from build123d import *

# Parameters (mm, degrees)
SKETCH1_R           = 9.25
SKETCH1_R_2         = 6.5
BOSS_EXTRUDE1_DEPTH = 62.5
BOSS_EXTRUDE2_START = -15
SKETCH3_R           = 12.5
SKETCH3_R_2         = 6.5
BOSS_EXTRUDE2_DEPTH = 15
BOSS_EXTRUDE3_START = 2.51
SKETCH4_R           = 9.25
SKETCH4_R_2         = 6.5
BOSS_EXTRUDE3_DEPTH = 2.51
BOSS_EXTRUDE4_START = 2.51
SKETCH5_R           = 12.5
SKETCH5_R_2         = 9.25
BOSS_EXTRUDE4_DEPTH = 2.51
CUT_EXTRUDE1_START  = -2.51
SKETCH6_R           = 12.5
SKETCH6_R_2         = 6.5
CUT_EXTRUDE1_DEPTH  = 2.51


with BuildPart() as part:
    # Sketch1 → Boss-Extrude1 (new body)
    with BuildSketch(Plane(origin=(0, 0, 0), x_dir=(1, 0, 0), z_dir=(0, 1, 0))):
        with Locations(Location((0, 0, 0), (0, 0, 270))):
            Circle(SKETCH1_R)
        with Locations(Location((0, 0, 0), (0, 0, 270))):
            Circle(SKETCH1_R_2, mode=Mode.SUBTRACT)
    extrude(amount=BOSS_EXTRUDE1_DEPTH)

    # Sketch3 → Boss-Extrude2 (add)
    with BuildSketch(Plane(origin=(0, 62.5, 0), x_dir=(1, 0, 0), z_dir=(0, 1, 0)).offset(BOSS_EXTRUDE2_START)):
        with Locations(Location((0, 0, 0), (0, 0, 270))):
            Circle(SKETCH3_R)
        with Locations(Location((0, 0, 0), (0, 0, 270))):
            Circle(SKETCH3_R_2, mode=Mode.SUBTRACT)
    extrude(amount=BOSS_EXTRUDE2_DEPTH)

    # Sketch4 → Boss-Extrude3 (add)
    with BuildSketch(Plane.XZ.offset(BOSS_EXTRUDE3_START)):
        with Locations(Location((0, 0, 0), (0, 0, 270))):
            Circle(SKETCH4_R)
        with Locations(Location((0, 0, 0), (0, 0, 270))):
            Circle(SKETCH4_R_2, mode=Mode.SUBTRACT)
    extrude(amount=-BOSS_EXTRUDE3_DEPTH)

    # Sketch5 → Boss-Extrude4 (add)
    with BuildSketch(Plane.XZ.offset(-47.5).offset(BOSS_EXTRUDE4_START)):
        with Locations(Location((0, 0, 0), (0, 0, 90))):
            Circle(SKETCH5_R)
        with Locations(Location((0, 0, 0), (0, 0, 270))):
            Circle(SKETCH5_R_2, mode=Mode.SUBTRACT)
    extrude(amount=-BOSS_EXTRUDE4_DEPTH)

    # Sketch6 → Cut-Extrude1 (cut)
    with BuildSketch(Plane(origin=(0, 62.5, 0), x_dir=(1, 0, 0), z_dir=(0, 1, 0)).offset(CUT_EXTRUDE1_START)):
        with Locations(Location((0, 0, 0), (0, 0, 270))):
            Circle(SKETCH6_R)
        with Locations(Location((0, 0, 0), (0, 0, 90))):
            Circle(SKETCH6_R_2, mode=Mode.SUBTRACT)
    extrude(amount=CUT_EXTRUDE1_DEPTH, mode=Mode.SUBTRACT)


solid = part.part
Build history of the part. All positions in model axes, mm. A direction names the side the tool comes from. Round coordinates to 2 decimals unless told otherwise and drop trailing zeros. Loops run counter-clockwise (first coordinate to the right, second up) from the corner with the lowest first, then second, coordinate; pieces in that order, holes last. Notation, with made-up numbers: (-29, 65.5) -> (-25, 65.5) arc R27 cw to (-25, 87.5) -> close; hole circle Ø5 at (39, 36.5). An arc over 180 degrees is marked (long way). One line per item, written item: value. Start each with the question number.
Q1. Probe line 1 along Z through (x, y) = (0, 34.5); line 2 along X through (y, z) = (50.5, -0.25). List the from-to ranges inside material, lowest first.
Q2. Cut at A-A on x = 0. List the corners of the cut face in (y, z), plus the area to 3 significant figures.
Q3. Drop flat-ended pins along their axis: pin 1 Ø12 at (y, z) = (8.5, -1.5) entering from +X; pin 2 Ø12 at (y, z) = (28, 0) entering from -X; pin 3 Ø8 at (x, y) = (-5.5, 12) entering from -Z. Give the stop position or say it passes through.
Q4. Cut at D-D on z = 8.5. List the corners of the cut face in (x, y), plus the area to 3 significant figures.
Q5. Cut at C-C on x = -7.25. List the corners of the cut face in (y, z), plus the area to 3 significant figures.
Q6. 3-axis set-ups, long thin cutter, end or side, ignore diameter. For faces 1 (the face through (-9.3, 44.99, 1.8)), 2 (the face through (-5, 59.99, 5)): which of +Z, -Z, +X, -X, +Y, -Y reach the whole face in a straight line?
Q7. Cut at B-B on z = -5. List the corners of the cut face in (x, y).
Computed:
1. line 1: -9.25 to -6.5, 6.5 to 9.25
1. line 2: -12.5 to -6.5, 6.5 to 12.5
2. outline: (-2.51, -9.25) -> (44.99, -9.25) -> (44.99, -12.5) -> (59.99, -12.5) -> (59.99, -6.5) -> (-2.51, -6.5) -> close; (-2.51, 6.5) -> (59.99, 6.5) -> (59.99, 12.5) -> (44.99, 12.5) -> (44.99, 9.25) -> (-2.51, 9.25) -> close
2. area: 441 mm²
3. pin 1: x = 9.25
3. pin 2: x = -9.25
3. pin 3: z = -9.13
4. outline: (-9.17, 44.99) -> (-3.65, 44.99) -> (-3.65, -2.51) -> (3.65, -2.51) -> (3.65, 44.99) -> (9.17, 44.99) -> (9.17, 59.99) -> (-9.17, 59.99) -> close
4. area: 622 mm²
5. outline: (-2.51, -5.74) -> (44.99, -5.74) -> (44.99, -10.18) -> (59.99, -10.18) -> (59.99, 10.18) -> (44.99, 10.18) -> (44.99, 5.74) -> (-2.51, 5.74) -> close
5. area: 851 mm²
6. face 1: -Y
6. face 2: +Z, -Z, +X, -X, +Y
7. outline: (-11.46, 44.99) -> (-7.78, 44.99) -> (-7.78, -2.51) -> (-4.15, -2.51) -> (-4.15, 59.99) -> (-11.46, 59.99) -> close; (4.15, -2.51) -> (7.78, -2.51) -> (7.78, 44.99) -> (11.46, 44.99) -> (11.46, 59.99) -> (4.15, 59.99) -> close
